Can you work these out from the model? Positions are in its coordinate system, mm. Face numbers are marked on the shaded views. A direction names the side the tool comes from. Coordinates: 2 decimals unless noted, no trailing zeros. Order: outer loops, then holes, each group sorted by start corner. A loop starts at its lowest first (then second) coordinate and runs counter-clockwise, first axis right, second up. Notation, with made-up numbers: (-17, 63.5) -> (28, 63.5) arc R23 cw to (28, 87.5) -> close; hole circle Ø3 at (-30.5, -4). An arc over 180 degrees is marked (long way). Use a Markdown table: item, result. Add a question column.
1. Suppose I cut it at B-B, the plane x = 274. List the corners of the cut face in (y, z) for me (3 decimals).
2. For the marked faces 1, 2 and 3, which set-ups out of +Z, -Z, +X, -X, +Y, -Y let a thin tool reach every point of the face, with its end or its side?
3. If I drill on line 1 along X through (y, z) = (-325, 41) (3 decimals); line 2 along Y through (x, z) = (-118, 39) (3 decimals); line 3 along Z through (x, y) = (312, -607) (3 decimals), over which ranges is the centre line in solid material (lowest first)? Write a range as from..to.
4. We'd pull the mould along X, two halves only. Please class the marked faces 4, 5, 6 and 7: pulls with the +X half, pulls with the -X half, needs draft (parallel to the pull), parting line crosses it, or undercut.
5. Suppose I cut it at A-A, the plane z = -51. List the corners of the cut face in (x, y) for me (3 decimals).
6. For pin 1 Ø2 at (x, z) = (205, -45.5) entering from +Y; pin 2 Ø5 at (x, y) = (-108, -522.5) entering from +Z (3 decimals); pin 3 Ø1 at (x, y) = (-291, -305.5) entering from -Z, each with a flat end and sliding along its axis, tell me the tip position at first contact or that it passes through.
7. Suppose I cut it at C-C, the plane y = -271. List the corners of the cut face in (x, z) for me (3 decimals).
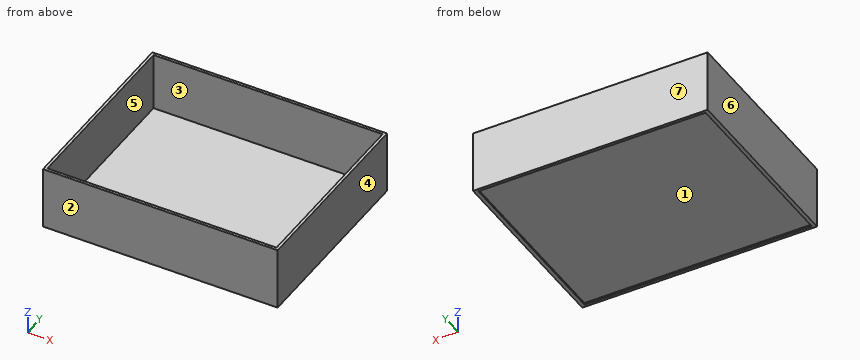
```python
from build123d import *

# Parameters (mm, degrees)
F0_W     = 806.45
F0_H     = 215.9
F1_DEPTH = 660.4
F2_W     = 781.05
F2_H     = 641.35
F3_DEPTH = 6.35
F4_T     = -9.525


# Not quite as in the source:
# - a shell that OpenCascade refuses in one call is made with other operations: the cavity is built on its own and cut out


with BuildPart() as f1:
    # F0 (on Front) → F1 (new body)
    with BuildSketch(Plane.XZ):
        Rectangle(F0_W, F0_H)
    extrude(amount=F1_DEPTH)

    # F2 (on face) → F3 (cut)
    with BuildSketch(Plane(origin=(0, 0, -107.95), x_dir=(1, 0, 0), z_dir=(0, 0, -1))):
        with Locations((0, 330.2)):
            Rectangle(F2_W, F2_H)
    extrude(amount=-F3_DEPTH, mode=Mode.SUBTRACT)

    # F4: a shell. OpenCascade refuses it in one call, so the cavity is built on its own and cut out:
    # the body offset inwards by the wall thickness, plus a prism from it out through each open face.
    f4_core = offset(f1.part, amount=F4_T, kind=Kind.INTERSECTION, mode=Mode.PRIVATE)
    f4_exits = [f4_core.faces().sort_by_distance(p)[0] for p in [
        (0, -330.2, 98.425),
    ]]
    add(f4_core, mode=Mode.SUBTRACT)
    extrude(f4_exits, amount=-F4_T, mode=Mode.SUBTRACT)


solid = f1.part
```
Worked out:
| question | item | result |
|---|---|---|
| 1 | outline | (-660.4, -107.95) -> (-650.875, -107.95) -> (-650.875, -101.6) -> (-9.525, -101.6) -> (-9.525, -107.95) -> (0, -107.95) -> (0, 107.95) -> (-9.525, 107.95) -> (-9.525, -92.075) -> (-650.875, -92.075) -> (-650.875, 107.95) -> (-660.4, 107.95) -> close |
| 2 | face 1 | -Z |
| 2 | face 2 | +Z, -Z, +X, -X, -Y |
| 2 | face 3 | +Z |
| 3 | line 1 | x = -403.225..-393.7, 393.7..403.225 |
| 3 | line 2 | y = -660.4..-650.875, -9.525..0 |
| 3 | line 3 | z = -101.6..-92.075 |
| 4 | face 4 | pulls with the +X half |
| 4 | face 5 | undercut |
| 4 | face 6 | pulls with the -X half |
| 4 | face 7 | needs draft |
| 5 | outline | (-403.225, -660.4) -> (403.225, -660.4) -> (403.225, 0) -> (-403.225, 0) -> close; hole (-393.7, -650.875) -> (393.7, -650.875) -> (393.7, -9.525) -> (-393.7, -9.525) -> close |
| 6 | pin 1 | stops at y = 0 |
| 6 | pin 2 | stops at z = -92.075 |
| 6 | pin 3 | stops at z = -101.6 |
| 7 | outline | (-403.225, -107.95) -> (-390.525, -107.95) -> (-390.525, -101.6) -> (390.525, -101.6) -> (390.525, -107.95) -> (403.225, -107.95) -> (403.225, 107.95) -> (393.7, 107.95) -> (393.7, -92.075) -> (-393.7, -92.075) -> (-393.7, 107.95) -> (-403.225, 107.95) -> close |
